from build123d import *

# Parameters (mm, degrees)
ESBO_O1_R                = 2
ESBO_O1_R_2              = 2.1
RESSALTO_EXTRUS_O1_DEPTH = 6
ESBO_O3_R                = 1.5
CORTE_EXTRUS_O1_DEPTH    = 232.669186565


with BuildPart() as part:
    # Esboço1 → Ressalto-extrusão1 (new body)
    with BuildSketch(Plane(origin=(0, 6, 0), x_dir=(1, 0, 0), z_dir=(0, 1, 0))):
        with BuildLine():
            Line((-3.5, 98), (-3.5, 105))
            ThreePointArc((-3.5, 105), (-4.964466094, 108.535533906), (-8.5, 110))
            Line((-8.5, 110), (-106.547005384, 110))
            ThreePointArc((-106.547005384, 110), (-116.547005384, 107.320508076), (-123.867513459, 100))
            Line((-123.867513459, 100), (-159.951905284, 37.5))
            ThreePointArc((-159.951905284, 37.5), (-170, 0), (-159.951905284, -37.5))
            Line((-159.951905284, -37.5), (-112.451905284, -119.772413359))
            ThreePointArc((-112.451905284, -119.772413359), (-85, -147.224318643), (-47.5, -157.272413359))
            Line((-47.5, -157.272413359), (47.5, -157.272413359))
            ThreePointArc((47.5, -157.272413359), (85, -147.224318643), (112.451905284, -119.772413359))
            Line((112.451905284, -119.772413359), (159.951905284, -37.5))
            ThreePointArc((159.951905284, -37.5), (170, 0), (159.951905284, 37.5))
            Line((159.951905284, 37.5), (123.867513459, 100))
            ThreePointArc((123.867513459, 100), (116.547005384, 107.320508076), (106.547005384, 110))
            Line((106.547005384, 110), (8.5, 110))
            ThreePointArc((8.5, 110), (4.964466094, 108.535533906), (3.5, 105))
            Line((3.5, 105), (3.5, 98))
            ThreePointArc((3.5, 98), (4.964466094, 94.464466094), (8.5, 93))
            Line((8.5, 93), (25, 93))
            ThreePointArc((25, 93), (28.535533906, 91.535533906), (30, 88))
            Line((30, 88), (30, 84))
            ThreePointArc((30, 84), (28.535533906, 80.464466094), (25, 79))
            Line((25, 79), (-25, 79))
            ThreePointArc((-25, 79), (-28.535533906, 80.464466094), (-30, 84))
            Line((-30, 84), (-30, 88))
            ThreePointArc((-30, 88), (-28.535533906, 91.535533906), (-25, 93))
            Line((-25, 93), (-8.5, 93))
            ThreePointArc((-8.5, 93), (-4.964466094, 94.464466094), (-3.5, 98))
        make_face()
        with Locations(Location((-82, -120, 0), (0, 0, 90))):
            Circle(ESBO_O1_R, mode=Mode.SUBTRACT)
        with Locations(Location((82, -120, 0), (0, 0, 90))):
            Circle(ESBO_O1_R, mode=Mode.SUBTRACT)
        with Locations(Location((150.5, -38.1, 0), (0, 0, 90))):
            Circle(ESBO_O1_R, mode=Mode.SUBTRACT)
        with Locations(Location((150.5, 38.1, 0), (0, 0, 90))):
            Circle(ESBO_O1_R, mode=Mode.SUBTRACT)
        with Locations(Location((-150.5, -38.1, 0), (0, 0, 90))):
            Circle(ESBO_O1_R, mode=Mode.SUBTRACT)
        with Locations(Location((-150.5, 38.1, 0), (0, 0, 90))):
            Circle(ESBO_O1_R, mode=Mode.SUBTRACT)
        with Locations(Location((15, 101.5, 0), (0, 0, 90))):
            Circle(ESBO_O1_R_2, mode=Mode.SUBTRACT)
        with Locations(Location((98, 102.4382, 0), (0, 0, 90))):
            Circle(ESBO_O1_R_2, mode=Mode.SUBTRACT)
        with Locations(Location((-15, 101.5, 0), (0, 0, 90))):
            Circle(ESBO_O1_R_2, mode=Mode.SUBTRACT)
        with Locations(Location((131.4, -57.5, 0), (0, 0, 90))):
            Circle(ESBO_O1_R, mode=Mode.SUBTRACT)
        with Locations(Location((-131.4, -57.5, 0), (0, 0, 90))):
            Circle(ESBO_O1_R, mode=Mode.SUBTRACT)
        with Locations(Location((131.4, 63, 0), (0, 0, 90))):
            Circle(ESBO_O1_R, mode=Mode.SUBTRACT)
        with Locations(Location((-131.4, 63, 0), (0, 0, 90))):
            Circle(ESBO_O1_R, mode=Mode.SUBTRACT)
        with Locations(Location((131.4, -70.2, 0), (0, 0, 90))):
            Circle(ESBO_O1_R, mode=Mode.SUBTRACT)
        with Locations(Location((-131.4, -70.2, 0), (0, 0, 90))):
            Circle(ESBO_O1_R, mode=Mode.SUBTRACT)
        with Locations(Location((131.4, 50.3, 0), (0, 0, 90))):
            Circle(ESBO_O1_R, mode=Mode.SUBTRACT)
        with Locations(Location((-131.4, 50.3, 0), (0, 0, 90))):
            Circle(ESBO_O1_R, mode=Mode.SUBTRACT)
        with Locations(Location((120, 55, 0), (0, 0, 90))):
            Circle(ESBO_O1_R_2, mode=Mode.SUBTRACT)
        with Locations(Location((-120, 55, 0), (0, 0, 90))):
            Circle(ESBO_O1_R_2, mode=Mode.SUBTRACT)
        with Locations(Location((-120, -55, 0), (0, 0, 90))):
            Circle(ESBO_O1_R_2, mode=Mode.SUBTRACT)
        with Locations(Location((120, -55, 0), (0, 0, 90))):
            Circle(ESBO_O1_R_2, mode=Mode.SUBTRACT)
        with Locations(Location((111.4552, 0, 0), (0, 0, 90))):
            Circle(ESBO_O1_R, mode=Mode.SUBTRACT)
        with Locations(Location((111.4552, 69.85, 0), (0, 0, 90))):
            Circle(ESBO_O1_R, mode=Mode.SUBTRACT)
        with Locations(Location((-111.4552, 0, 0), (0, 0, 90))):
            Circle(ESBO_O1_R, mode=Mode.SUBTRACT)
        with Locations(Location((-111.4552, 69.85, 0), (0, 0, 90))):
            Circle(ESBO_O1_R, mode=Mode.SUBTRACT)
        with Locations(Location((-97.9932, 0, 0), (0, 0, 90))):
            Circle(ESBO_O1_R, mode=Mode.SUBTRACT)
        with Locations(Location((97.9932, 0, 0), (0, 0, 90))):
            Circle(ESBO_O1_R, mode=Mode.SUBTRACT)
        with Locations(Location((0, 0, 0), (0, 0, 90))):
            Circle(ESBO_O1_R, mode=Mode.SUBTRACT)
        with Locations(Location((98, -109.22, 0), (0, 0, 90))):
            Circle(ESBO_O1_R_2, mode=Mode.SUBTRACT)
        with Locations(Location((-98, -109.22, 0), (0, 0, 90))):
            Circle(ESBO_O1_R_2, mode=Mode.SUBTRACT)
        with Locations(Location((0, -109.22, 0), (0, 0, 90))):
            Circle(ESBO_O1_R_2, mode=Mode.SUBTRACT)
        with Locations(Location((-98, 102.4382, 0), (0, 0, 90))):
            Circle(ESBO_O1_R_2, mode=Mode.SUBTRACT)
        with BuildLine():
            Line((123.22, 12), (123.22, -12))
            ThreePointArc((123.22, -12), (121.22, -14), (119.22, -12))
            Line((119.22, -12), (119.22, 12))
            ThreePointArc((119.22, 12), (121.22, 14), (123.22, 12))
        make_face(mode=Mode.SUBTRACT)
        with BuildLine():
            Line((-123.22, -12), (-123.22, 12))
            ThreePointArc((-123.22, 12), (-121.22, 14), (-119.22, 12))
            Line((-119.22, 12), (-119.22, -12))
            ThreePointArc((-119.22, -12), (-121.22, -14), (-123.22, -12))
        make_face(mode=Mode.SUBTRACT)
    extrude(amount=-RESSALTO_EXTRUS_O1_DEPTH)

    # Esboço3 → Corte-extrusão1 (cut, through all)
    with BuildSketch(Plane(origin=(0, 6, 0), x_dir=(1, 0, 0), z_dir=(0, 1, 0))):
        with Locations(Location((-57.15, -143.272413359, 0), (0, 0, 270))):
            Circle(ESBO_O3_R)
        with Locations(Location((57.15, -143.272413359, 0), (0, 0, 270))):
            Circle(ESBO_O3_R)
        with Locations(Location((-57.15, -124.222413359, 0), (0, 0, 270))):
            Circle(ESBO_O3_R)
        with Locations(Location((57.15, -124.222413359, 0), (0, 0, 270))):
            Circle(ESBO_O3_R)
        with Locations(Location((-57.15, -105.172413359, 0), (0, 0, 270))):
            Circle(ESBO_O3_R)
        with Locations(Location((57.15, -105.172413359, 0), (0, 0, 270))):
            Circle(ESBO_O3_R)
    extrude(amount=-CORTE_EXTRUS_O1_DEPTH, mode=Mode.SUBTRACT)


solid = part.part
Source: CAD feature listing. Evaluate the final solid. Frame: model axes, mm. Round coordinates to 2 decimals unless told otherwise and drop trailing zeros. Write each loop counter-clockwise with the first axis right and the second up, starting at its lowest first coordinate (ties: lowest second). Pieces come first, ordered by that corner, then holes. Notation, with made-up numbers: (-25, 1.25) - (21, 1.25) arc R16 ccw to (21, 18.25) - close; hole circle Ø8 at (32, 1). An arc over 180 degrees is marked (long way). Use CSV: the item, a comma, the result in double quotes. Start each with the question number.
(1) Cut plane B-B, the plane z = 31. Return loops of the section in (x, y).
(2) Material intervals for probe 1 along Z at (x, y) = (-10, 4.35); probe 2 along X at (y, z) = (4.85, 37); probe 3 along Z at (x, y) = (-150.5, 2.55), sorted ascending. Write a range as [from, to].
(3) Cut plane A-A, the plane y = 2. Give the number of separate pieces and of enclosed holes in the cut face, and give its area (3 significant figures).
(4) First-contact query: pin 1 Ø1 at (x, y) = (71, 1) entering from +Z; pin 2 Ø6.5 at (x, z) = (-120, 55) entering from +Y; pin 3 Ø2 at (y, z) = (5, -3.5) entering from +X; pin 4 Ø1.5 at (y, z) = (5, -15) entering from -X. Flat tips, straight axial feed; report the tip coordinate or a pass-through.
Geometry says:
1,outline,"(-163.29, 0) - (163.29, 0) - (163.29, 6) - (-163.29, 6) - close"
2,probe 1,"[-110, -93], [-79, 157.27]"
2,probe 2,"[-160.24, -152.17], [-148.83, 148.83], [152.17, 160.24]"
2,probe 3,"[-53.87, -40.1], [-36.1, 36.1], [40.1, 53.87]"
3,separate pieces,"1"
3,enclosed holes,"40"
3,area,"72,900 mm²"
4,pin 1,"z = 153.66"
4,pin 2,"y = 6"
4,pin 3,"x = 169.96"
4,pin 4,"x = -168.63"
